Read the model definition and answer for the solid it produces. Units are mm, in the model's axes. A direction names the side the tool comes from. Give positions to 0.01 mm unless a question says otherwise; leave off trailing zeros. Write each loop counter-clockwise with the first axis right and the second up, starting at its lowest first coordinate (ties: lowest second). Pieces come first, ordered by that corner, then holes. Notation, with made-up numbers: M -24.5,10 L 3.5,10 A21 ccw 3.5,28 Z; hole C 18,39.5 d2. An arc over 180 degrees is marked long. Use a Markdown table: item, result. Add a question column.
Item 1: A cutting plane is placed at B-B on x = 16. Determine the outline of the cut face in (y, z).
Item 2: The mould has two halves that part along Z. Classify faces 1 (the flat face through (-40, 0, 12)), 2 (the flat face through (-47.606, 172.55, 11.914)), 3 (the cylindrical face through (-71.935, 172.55, 4.281)): pulls with the +Z half, pulls with the -Z half, needs draft (parallel to the pull), parting line crosses it, or undercut.
Item 3: Consider probe 1 along Z at (x, y) = (-17.5, 244); probe 2 along Z at (x, y) = (-65.5, 136); probe 3 along Z at (x, y) = (-35, 298.5). Determine where each line is inside the solid, lowest interval first. Write a range as [from, to].
Item 4: Given P1, Ø0.8, axis at x = -6.5, z = 0.5, coming from the -Y side; P2, Ø1, axis at y = 82, z = 3, coming from the +X side; P3, Ø4, axis at y = 99.5, z = 1, coming from the -X side; P4, Ø7, axis at x = 39, z = 6.5, coming from the -Y side, each flat-ended and moving along its own axis, determine where each tip first touches the part or whether it passes through.
Item 5: A cutting plane is placed at A-A on y = 206. Determine the outline of the cut face in (x, z).
Item 6: For faces 4 (the cylindrical face through (-72.96, 172.55, 4.36)), 5 (the flat face through (-26.25, 173, 7)), 6 (the flat face through (-22.25, 173, 7)), 7 (the flat face through (22.25, -50, -2)), 8 (the flat face through (68, -50, -2)), determine the directions among +Z, -Z, +X, -X, +Y, -Y from which every point of the face is accessible in a straight line to the end or side of a thin tool.
from build123d import *

# Parameters (mm, degrees)
F1_DEPTH = 350
F4_DEPTH = 45.75


with BuildPart() as f1:
    # F0 (on Front) → F1 (new body)
    with BuildSketch(Plane.XZ):
        with BuildLine():
            ThreePointArc((-69.4691266018, 9.7792956623), (-72.9445160689, 4.257193939), (-68, 0))
            Line((-68, 0), (0, 0))
            Line((0, 0), (68, 0))
            ThreePointArc((68, 0), (72.9445160689, 4.257193939), (69.4691266018, 9.7792956623))
            Line((69.4691266018, 9.7792956623), (26.3469652224, 13.9905305459))
            ThreePointArc((26.3469652224, 13.9905305459), (26.2498846097, 13.9976312337), (26.1525734896, 14))
            Line((26.1525734896, 14), (26.0150079844, 14))
            Line((26.0150079844, 14), (22.25, 14))
            Line((22.25, 14), (22.25, 1))
            Line((22.25, 1), (0, 1))
            Line((0, 1), (-22.25, 1))
            Line((-22.25, 1), (-22.25, 14))
            Line((-22.25, 14), (-26.0150079844, 14))
            Line((-26.0150079844, 14), (-26.1525734896, 14))
            ThreePointArc((-26.1525734896, 14), (-26.2498846097, 13.9976312337), (-26.3469652224, 13.9905305459))
            Line((-26.3469652224, 13.9905305459), (-69.4691266018, 9.7792956623))
        make_face()
        with BuildLine():
            Line((-26.25, 12.9720028672), (-26.25, 1))
            Line((-26.25, 1), (-68, 1))
            ThreePointArc((-68, 1), (-71.9482597731, 4.3587163152), (-69.265977288, 8.7943776178))
            Line((-69.265977288, 8.7943776178), (-26.25, 12.9952427487))
            Line((-26.25, 12.9952427487), (-26.25, 12.9720028672))
        make_face(mode=Mode.SUBTRACT)
        with BuildLine():
            Line((68, 1), (26.25, 1))
            Line((26.25, 1), (26.25, 12.9720028672))
            Line((26.25, 12.9720028672), (26.25, 12.9952427487))
            Line((26.25, 12.9952427487), (69.265977288, 8.7943776178))
            ThreePointArc((69.265977288, 8.7943776178), (71.9482597731, 4.3587163152), (68, 1))
        make_face(mode=Mode.SUBTRACT)
    extrude(amount=-F1_DEPTH)

    # F3 (on offset) → F4 (join)
    with BuildSketch(Plane.YZ.offset(-22.25)):
        with BuildLine():
            add(Edge.make_bspline(
                [(0, 0), (-36.9747690856, 0), (-56.282736361, 0), (-100.0474691391, -14.7872483358)],
                knots=[0, 0, 0, 0, 101.1343601081, 101.1343601081, 101.1343601081, 101.1343601081], degree=3))
            Line((0, 0), (0, 1))
            add(Edge.make_bspline(
                [(0, 1), (-9.2436922714, 1), (-25.5401100661, 1.0005275684), (-47.3845795682, -0.3908549289), (-70.5242758511, -4.5730687745), (-89.4052629561, -10.135915446), (-100.3675713535, -13.8398653233)],
                knots=[0, 0, 0, 0, 0.25, 0.5, 0.75, 1, 1, 1, 1], degree=3))
            Line((-100.3675713535, -13.8398653233), (-100.0474691391, -14.7872483358))
        make_face()
    extrude(amount=-F4_DEPTH)

    # F5: F1 across plane


with BuildPart() as f1_1:
    add(f1.part)
    add(f1.part.mirror(Plane.YZ))


solid = f1_1.part
Filled in:
| question | item | result |
|---|---|---|
| 1 | outline | M 0,0 L 350,0 L 350,1 L 0,1 Z |
| 2 | face 1 | needs draft |
| 2 | face 2 | pulls with the +Z half |
| 2 | face 3 | undercut |
| 3 | probe 1 | [0, 1] |
| 3 | probe 2 | [0, 1], [9.16, 10.17] |
| 3 | probe 3 | [0, 1], [12.14, 13.15] |
| 4 | P1 | y = 0 |
| 4 | P2 | x = 72.77 |
| 4 | P3 | x = -72.58 |
| 4 | P4 | through |
| 5 | outline | M -69.47,9.78 A5 ccw -68,0 L 68,0 A5 ccw 69.47,9.78 L 26.35,13.99 A2 ccw 26.15,14 L 22.25,14 L 22.25,1 L -22.25,1 L -22.25,14 L -26.15,14 A2 ccw -26.35,13.99 Z; hole M -69.27,8.79 A4 ccw -68,1 L -26.25,1 L -26.25,13 Z; hole M 26.25,1 L 68,1 A4 ccw 69.27,8.79 L 26.25,13 Z |
| 6 | face 4 | -X, +Y, -Y |
| 6 | face 5 | +Y, -Y |
| 6 | face 6 | +Z, +Y, -Y |
| 6 | face 7 | +Z, -Z, -Y |
| 6 | face 8 | +Z, -Z, +X, -Y |
